The listing builds one solid part. Answer for the finished solid, in the listing's coordinates (mm). A direction names the side the tool comes from. Coordinates: 2 decimals unless noted, no trailing zeros. Loops run counter-clockwise (first coordinate to the right, second up) from the corner with the lowest first, then second, coordinate; pieces in that order, holes last. Notation, with made-up numbers: (18, 46.5) - (46, 46.5) arc R15 cw to (46, 51.5) - close; hole circle Ø5 at (-28.5, 19.5). An arc over 180 degrees is marked (long way). Write each question's results on one line, items separated by ' | '. Start each with the question number.
(1) Consider line 1 (X direction, y = -25.4, z = -2.75); line 2 (Y direction, x = 14, z = -3.25); line 3 (Y direction, x = -194, z = -14.5). Determine where each line is inside the solid, lowest interval first. Write a range as from..to.
(2) Find section A-A on y = -230. Determine the outline of the cut face in (x, z), then the cut area to 3 significant figures.
(3) For faces 1 (the flat face through (15, -384, 0)), 2 (the flat face through (12.7, -198, -9)), determine the directions among +Z, -Z, +X, -X, +Y, -Y from which every point of the face is accessible in a straight line to the end or side of a thin tool.
(4) Determine the mould class of faces 3 (the flat face through (-196.65, -591.88, -9.39)), 4 (the cylindrical face through (27.473, -435.929, -9.392)), 5 (the flat face through (-254.24, -521.4, -9.39)) for opening direction X: released by +X, released by -X, zero draft, split by the parting line, or undercut.
(5) Find section B-B on y = -434. Determine the outline of the cut face in (x, z), then the cut area to 3 significant figures.
(6) Given pin 1 Ø3.5 at (y, z) = (-75.31, -9.53) entering from +X; pin 2 Ø6 at (y, z) = (-439.5, -4.5) entering from +X; pin 3 Ø2 at (y, z) = (-354, -10) entering from -X, each flat-ended and moving along its own axis, determine where each tip first touches the part or whether it passes through.
from build123d import *

# Parameters (mm, degrees)
BOSS_EXTRUDE1_DEPTH = 19.05
CHAMFER1_SIZE       = 25.4
CHAMFER1_SIZE2      = 23.3906272
HOLE2_D             = 3.175
HOLE2_DEPTH         = 31.75
HOLE2_CSINK_D       = 10.16
HOLE2_CSINK_ANGLE   = 82
HOLE2_TIP           = 0.953866233
HOLE4_D             = 3.175
HOLE4_DEPTH         = 31.75
HOLE4_CSINK_D       = 10.16
HOLE4_CSINK_ANGLE   = 82
HOLE4_TIP           = 0.953866233
HOLE5_D             = 3.175
HOLE5_DEPTH         = 38.1
HOLE5_CSINK_D       = 10.16
HOLE5_CSINK_ANGLE   = 82
HOLE5_TIP           = 0.953866233
HOLE6_D             = 3.175
HOLE6_DEPTH         = 38.1
HOLE6_CSINK_D       = 10.16
HOLE6_CSINK_ANGLE   = 82
HOLE6_TIP           = 0.953866233


with BuildPart() as part:
    # Sketch1 → Boss-Extrude1 (new body)
    with BuildSketch(Plane.XY):
        with BuildLine():
            Line((12.7, 12.7), (12.7, -415.185594934))
            ThreePointArc((12.7, -415.185594934), (27.339445595, -436.32629993), (2.687239133, -443.641454859))
            Line((2.687239133, -443.641454859), (-518.461959982, -601.369999539))
            Line((-518.461959982, -601.369999539), (-494.089021628, -681.900364725))
            Line((-494.089021628, -681.900364725), (109.245636646, -499.2979588))
            Line((109.245636646, -499.2979588), (155.492294041, 12.7))
            Line((155.492294041, 12.7), (12.7, 12.7))
        make_face()
    extrude(amount=-BOSS_EXTRUDE1_DEPTH)

    # Chamfer1
    chamfer1_edges = [part.edges().sort_by_distance(p)[0] for p in [
        (155.492294041, 12.7, -9.525),
    ]]
    chamfer1_side = [part.faces().sort_by_distance(p)[0] for p in [
        (84.09614702, 12.7, -9.525),
    ]]
    chamfer(chamfer1_edges, length=CHAMFER1_SIZE, length2=CHAMFER1_SIZE2, reference=chamfer1_side[0])

    # Hole2
    with Locations(Plane(origin=(0, 10.424290059, 165.474999994), x_dir=(0, 0, -1), z_dir=(-1, 0, 0))):
        with Locations((-155.949999994, 107.734820482), (155.949999994, 107.734820482), (155.949999994, 327.755881328), (174.999999994, 85.732714397), (174.999999994, 349.757987412), (-174.999999994, 349.757987412), (-174.999999994, 85.732714397), (-155.949999994, 327.755881328)):
            CounterSinkHole(HOLE2_D / 2, HOLE2_CSINK_D / 2, depth=HOLE2_DEPTH, counter_sink_angle=HOLE2_CSINK_ANGLE)
            with Locations((0, 0, -(HOLE2_DEPTH + HOLE2_TIP / 2))):  # 118° drill point
                Cone(0, HOLE2_D / 2, HOLE2_TIP, mode=Mode.SUBTRACT)

    # Hole4
    with Locations(Plane(origin=(264.696145853, -351.074163461, 165.474999994), x_dir=(0, 0, -1), z_dir=(-0.2896786029738453, 0.9571239768071436, 8.258871730585588e-15))):
        with Locations((174.999999994, 685.961004241), (174.999999994, 549.837259632), (174.999999994, 413.713515022), (81.549999997, 779.649723129), (81.549999997, 652.344645962), (62.499999997, 662.953402392), (62.499999997, 769.040966698), (-62.499999997, 769.040966698), (-62.499999997, 662.953402392), (-81.549999997, 652.344645962), (-81.549999997, 779.649723129), (-174.999999994, 413.713515022), (-174.999999994, 549.837259632), (-174.999999994, 685.961004241), (-82.737499997, 600.384620239), (0, 600.384620239), (82.737499997, 600.384620239), (0, 376.737770337), (-82.737499997, 376.737770337), (82.737499997, 376.737770337)):
            CounterSinkHole(HOLE4_D / 2, HOLE4_CSINK_D / 2, depth=HOLE4_DEPTH, counter_sink_angle=HOLE4_CSINK_ANGLE)
            with Locations((0, 0, -(HOLE4_DEPTH + HOLE4_TIP / 2))):  # 118° drill point
                Cone(0, HOLE4_D / 2, HOLE4_TIP, mode=Mode.SUBTRACT)

    # Hole5
    with Locations(Plane(origin=(155.286738577, 10.424290059, -19.05), x_dir=(-0.08995962873759064, -0.9959454127598535, 0), z_dir=(0, 0, -1))):
        with Locations((46.221112845, 113.488854888), (39.39759596, 37.945520226), (412.28786892, 80.423559293), (407.308516105, 25.297013484), (513.561319184, 161.164706775), (597.46020397, 127.267357003), (610.543339245, 159.649253123), (694.322923815, 367.011001477), (526.644454459, 193.546602895), (610.424039029, 400.908351249)):
            CounterSinkHole(HOLE5_D / 2, HOLE5_CSINK_D / 2, depth=HOLE5_DEPTH, counter_sink_angle=HOLE5_CSINK_ANGLE)
            with Locations((0, 0, -(HOLE5_DEPTH + HOLE5_TIP / 2))):  # 118° drill point
                Cone(0, HOLE5_D / 2, HOLE5_TIP, mode=Mode.SUBTRACT)

    # Hole6
    with Locations(Plane(origin=(-643.705760022, -231.394989772, 165.474999994), x_dir=(0, 0, -1), z_dir=(-0.9571239768071421, -0.2896786029738502, -1.2569443472852944e-15))):
        with Locations((-108.649999997, 332.89193461), (108.649999997, 332.89193461), (207.774999994, 332.89193461), (174.999999994, 448.336332751), (135.266666663, 384.042401694), (176.283333328, 384.042401694), (-174.999999994, 448.336332751), (-135.266666663, 384.042401694), (-176.283333328, 384.042401694), (-207.774999994, 332.89193461)):
            CounterSinkHole(HOLE6_D / 2, HOLE6_CSINK_D / 2, depth=HOLE6_DEPTH, counter_sink_angle=HOLE6_CSINK_ANGLE)
            with Locations((0, 0, -(HOLE6_DEPTH + HOLE6_TIP / 2))):  # 118° drill point
                Cone(0, HOLE6_D / 2, HOLE6_TIP, mode=Mode.SUBTRACT)


solid = part.part
Values:
1) line 1: x = 12.7..36.51, 39.69..112.36, 115.54..152.05 | line 2: y = -528.12..-446.85, -415.27..12.7 | line 3: y = -591.08..-503.17
2) outline: (12.7, -19.05) - (133.57, -19.05) - (133.57, 0) - (12.7, 0) - close | area: 2,300 mm²
3) face 1: +Z, +X, -X, +Y, -Y | face 2: +Z, -Z, -X, +Y
4) face 3: released by +X | face 4: undercut | face 5: released by -X
5) outline: (27.96, -19.05) - (115.14, -19.05) - (115.14, 0) - (27.96, 0) - close | area: 1,660 mm²
6) pin 1: stops at x = 147.7 | pin 2: stops at x = 114.92 | pin 3: stops at x = 12.7
